```python
from build123d import *

# Parameters (mm, degrees)
SKETCH_W        = 200
SKETCH_H        = 17.7
SKETCH_R        = 1.2
PAD_DEPTH       = 10
SKETCH001_R     = 2.1
POCKET_DEPTH    = 3.3
SKETCH002_W     = 7
SKETCH002_H     = 1
POCKET001_DEPTH = 200
SKETCH012_W     = 5
SKETCH012_H     = 5
PAD003_DEPTH    = 1.5
SKETCH013_W     = 1
SKETCH013_H     = 6
POCKET009_DEPTH = 200


with BuildPart() as part:
    # Sketch → Pad (new body)
    with BuildSketch(Plane.XY):
        Rectangle(SKETCH_W, SKETCH_H)
        with Locations((-75, 0)):
            Circle(SKETCH_R, mode=Mode.SUBTRACT)
        with Locations((-15, 0)):
            Circle(SKETCH_R, mode=Mode.SUBTRACT)
        with Locations((45, 0)):
            Circle(SKETCH_R, mode=Mode.SUBTRACT)
        with Locations((-94.96, 4)):
            Circle(SKETCH_R, mode=Mode.SUBTRACT)
        with Locations((-82.96, 4)):
            Circle(SKETCH_R, mode=Mode.SUBTRACT)
        with Locations((-94.96, -4)):
            Circle(SKETCH_R, mode=Mode.SUBTRACT)
        with Locations((-82.96, -4)):
            Circle(SKETCH_R, mode=Mode.SUBTRACT)
        with Locations((82.96, 4)):
            Circle(SKETCH_R, mode=Mode.SUBTRACT)
        with Locations((94.96, 4)):
            Circle(SKETCH_R, mode=Mode.SUBTRACT)
        with Locations((82.96, -4)):
            Circle(SKETCH_R, mode=Mode.SUBTRACT)
        with Locations((94.96, -4)):
            Circle(SKETCH_R, mode=Mode.SUBTRACT)
    extrude(amount=PAD_DEPTH)

    # Sketch001 (on Face17 of Pad) → Pocket (cut)
    with BuildSketch(Plane.XY.offset(10)):
        with Locations((94.96, -4)):
            Circle(SKETCH001_R)
        with Locations((-94.96, 4)):
            Circle(SKETCH001_R)
        with Locations((-82.96, 4)):
            Circle(SKETCH001_R)
        with Locations((-82.96, -4)):
            Circle(SKETCH001_R)
        with Locations((94.96, 4)):
            Circle(SKETCH001_R)
        with Locations((82.96, 4)):
            Circle(SKETCH001_R)
        with Locations((-94.96, -4)):
            Circle(SKETCH001_R)
        with Locations((82.96, -4)):
            Circle(SKETCH001_R)
    extrude(amount=-POCKET_DEPTH, mode=Mode.SUBTRACT)

    # Sketch002 (on Face3 of Pocket) → Pocket001 (cut)
    with BuildSketch(Plane.YZ.offset(100)):
        with Locations((0, 9.5)):
            Rectangle(SKETCH002_W, SKETCH002_H)
    extrude(amount=-POCKET001_DEPTH, mode=Mode.SUBTRACT)

    # Sketch012 (on Face9 of Pocket001) → Pad003 (join)
    with BuildSketch(Plane.XY.offset(10)):
        with Locations((88.75, 6.35)):
            Rectangle(SKETCH012_W, SKETCH012_H)
        with Locations((-88.75, 6.35)):
            Rectangle(SKETCH012_W, SKETCH012_H)
    extrude(amount=PAD003_DEPTH)

    # Sketch013 (on Face3 of Pad003) → Pocket009 (cut)
    with BuildSketch(Plane.YZ.offset(100)):
        with Locations((8.35, 5)):
            Rectangle(SKETCH013_W, SKETCH013_H)
    extrude(amount=-POCKET009_DEPTH, mode=Mode.SUBTRACT)


solid = part.part
```
Geometry: final body of the model. Coordinates: model frame, mm. A direction names the side the tool comes from. Round coordinates to 2 decimals unless told otherwise and drop trailing zeros. Write each loop counter-clockwise with the first axis right and the second up, starting at its lowest first coordinate (ties: lowest second). Pieces come first, ordered by that corner, then holes. Notation, with made-up numbers: (41.5, 67.25) -> (85.5, 67.25) arc R26 ccw to (85.5, 81.25) -> close; hole circle Ø4 at (-6, 72.5). An arc over 180 degrees is marked (long way). Use CSV: the item, a comma, the result in double quotes. Start each with the question number.
Q1. Line query: L1, parallel to Y at x = -94.96, z = 7.75; L2, parallel to X at y = 4, z = 8.8; L3, parallel to Y at x = 94.96, z = 2.5. Output: solid intervals per line, ascending.
Q2. Reachability of faces 1 (the face through (-89, 6, 11.5)), 2 (the face through (-95.233, 6.082, 8.006)) from +Z, -Z, +X, -X, +Y, -Y: full face, straight path, thin tool, end or side. Return the list, or none.
Q3. Section B-B (x = -43.5). Return loops of the section in (y, z).
Q4. Section A-A (z = 3.75). Give the number of separate pieces and of enclosed holes in the cut face, plus the area to 3 significant figures.
Q5. First-contact query: pin 1 Ø5.5 at (x, y) = (-94.96, 4) entering from -Z; pin 2 Ø1.3 at (x, y) = (82.5, 3.5) entering from +Z; pin 3 Ø2 at (x, y) = (-75, 0) entering from -Z; pin 4 Ø1.5 at (x, z) = (6, 3.5) entering from +Y. Flat tips, straight axial feed; report the tip coordinate or a pass-through.
Q6. Pull-direction query (X, two-part tool) for faces 3 (the face through (100, 0, 5)), 4 (the face through (94.5, -6.05, 8.01)), 5 (the face through (-1, -8.85, 5)); classes: pulls with the +X half, pulls with the -X half, needs draft (parallel to the pull), parting line crosses it, or undercut.
Result sheet:
1,L1,"-8.85 to -6.1, -1.9 to 1.9, 6.1 to 7.85"
1,L2,"-100 to -97.06, -92.86 to -85.06, -80.86 to 80.86, 85.06 to 92.86, 97.06 to 100"
1,L3,"-8.85 to -5.2, -2.8 to 2.8, 5.2 to 7.85"
2,face 1,"+Z, +X, -X, +Y, -Y"
2,face 2,"+Z"
3,outline,"(-8.85, 0) -> (8.85, 0) -> (8.85, 2) -> (7.85, 2) -> (7.85, 8) -> (8.85, 8) -> (8.85, 10) -> (3.5, 10) -> (3.5, 9) -> (-3.5, 9) -> (-3.5, 10) -> (-8.85, 10) -> close"
4,separate pieces,"1"
4,enclosed holes,"11"
4,area,"3,290 mm²"
5,pin 1,"z = 0"
5,pin 2,"z = 6.7"
5,pin 3,"through"
5,pin 4,"y = 7.85"
6,face 3,"pulls with the +X half"
6,face 4,"undercut"
6,face 5,"needs draft"
